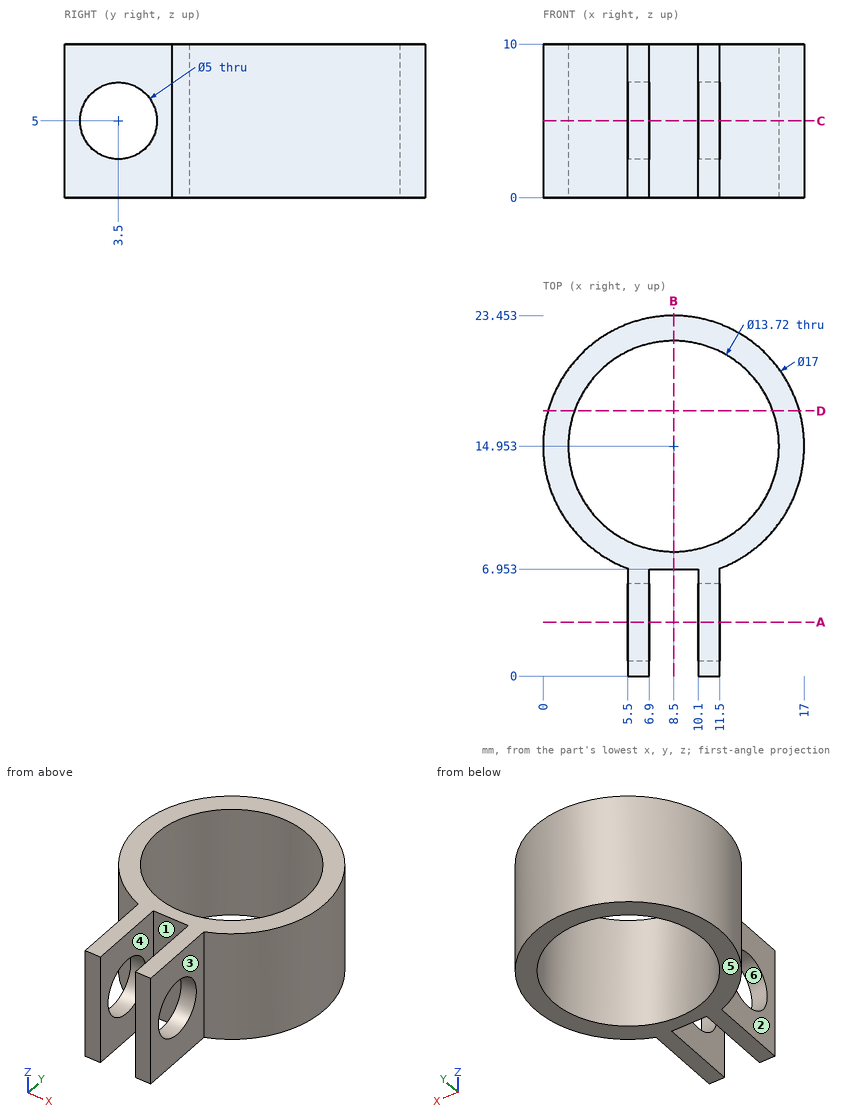
Design review of the part shown in the three views and the two pictorial views. Dimensions are in mm from the part's minimum x, y and z. A direction names the side the tool comes from. Coordinates: 2 decimals unless noted, no trailing zeros. Loops run counter-clockwise (first coordinate to the right, second up) from the corner with the lowest first, then second, coordinate; pieces in that order, holes last.
(1) Consider section D-D, the plane y = 17.25. Give the boundary of the cut face in (x, z), plus the area to 3 significant figures.
Determined:
outline: (0.32, 0) - (2.04, 0) - (2.04, 10) - (0.32, 10) - close; (14.96, 0) - (16.68, 0) - (16.68, 10) - (14.96, 10) - close
area: 34.4 mm2
(2) Consider section A-A, the plane y = 3.5. Give the boundary of the cut face in (x, z), plus the area to 3 significant figures.
Determined:
outline: (5.5, 0) - (6.9, 0) - (6.9, 2.5) - (5.5, 2.5) - close; (5.5, 7.5) - (6.9, 7.5) - (6.9, 10) - (5.5, 10) - close; (10.1, 0) - (11.5, 0) - (11.5, 2.5) - (10.1, 2.5) - close; (10.1, 7.5) - (11.5, 7.5) - (11.5, 10) - (10.1, 10) - close
area: 14.0 mm2
(3) Tool access review of the marked faces 1, 2 and 3: name each direction out of +Z, -Z, +X, -X, +Y, -Y from which nothing blocks a thin tool from reaching the whole face with its end or side.
Determined:
face 1: +Z, -Z, -Y
face 2: +Z, -Z, -X, -Y
face 3: +Z, -Z, +X, -Y
(4) Insertion check: P1, Ø5.5, axis at y = 3.5, z = 5, coming from the -X side; P2, Ø1, axis at y = 16.5, z = 7.5, coming from the +X side; P3, Ø2, axis at y = 18.5, z = 3.5, coming from the -X side. Each pin has a flat end and moves straight along its axis. Give the tip position at first contact, or say it passes through.
Determined:
P1: stops at x = 5.5
P2: stops at x = 16.94
P3: stops at x = 0.39
(5) Draft analysis for pull direction Z (two halves, no side actions). For the marked faces 4, 5 and 6, state which applies: +Z half, -Z half, draft (parallel to the pull), parting line (faces both ways), or undercut.
Determined:
face 4: draft
face 5: -Z half
face 6: undercut
(6) Consider section C-C, the plane z = 5. Give the boundary of the cut face in (x, y), plus the area to 3 significant figures.
Determined:
outline: (5.5, 0) - (6.9, 0) - (6.9, 1) - (5.5, 1) - close; (5.5, 6) - (6.9, 6) - (6.9, 6.95) - (10.1, 6.95) - (10.1, 6) - (11.5, 6) - (11.5, 7) arc R8.5 ccw (long way) to (5.5, 7) - close; (10.1, 0) - (11.5, 0) - (11.5, 1) - (10.1, 1) - close; hole circle Ø13.72 at (8.5, 14.95)
area: 82.7 mm2
(7) Consider section B-B, the plane x = 8.5. Give the boundary of the cut face in (y, z), plus the area to 3 significant figures.
Determined:
outline: (6.95, 0) - (8.09, 0) - (8.09, 10) - (6.95, 10) - close; (21.81, 0) - (23.45, 0) - (23.45, 10) - (21.81, 10) - close
area: 27.8 mm2
(8) Wall thickness on L1, parallel to Z at x = 5.9, y = 3.5; L2, parallel to X at y = 2.25, z = 9.5; L3, parallel to Y at x = 9.5, z = 1.75: over which ranges is each line inside the solid? List them lowest first.
Determined:
L1: z = 0 to 2.5, 7.5 to 10
L2: x = 5.5 to 6.9, 10.1 to 11.5
L3: y = 6.95 to 8.17, 21.74 to 23.39
